from build123d import *

# Parameters (mm, degrees)
SKETCH2_W           = 35
SKETCH2_H           = 10
BOSS_EXTRUDE1_DEPTH = 4
FILLET1_R           = 2
BOSS_EXTRUDE2_DEPTH = 13


with BuildPart() as part:
    # Sketch2 → Boss-Extrude1 (new body)
    with BuildSketch(Plane.XY):
        Rectangle(SKETCH2_W, SKETCH2_H)
    extrude(amount=BOSS_EXTRUDE1_DEPTH)

    # Fillet1
    fillet1_edges = [part.edges().sort_by_distance(p)[0] for p in [
        (17.5, -5, 2),
        (-17.5, -5, 2),
        (-17.5, 5, 2),
        (17.5, 5, 2),
    ]]
    fillet(fillet1_edges, radius=FILLET1_R)

    # Sketch3 → Boss-Extrude2 (add)
    with BuildSketch(Plane.XY.offset(4)):
        with BuildLine():
            Line((-16.5, 3), (-16.5, -3))
            ThreePointArc((-16.5, -3), (-16.207106781, -3.707106781), (-15.5, -4))
            Line((-15.5, -4), (15.5, -4))
            ThreePointArc((15.5, -4), (16.207106781, -3.707106781), (16.5, -3))
            Line((16.5, -3), (16.5, 3))
            ThreePointArc((16.5, 3), (16.207106781, 3.707106781), (15.5, 4))
            Line((15.5, 4), (-15.5, 4))
            ThreePointArc((-15.5, 4), (-16.207106781, 3.707106781), (-16.5, 3))
        make_face()
    extrude(amount=BOSS_EXTRUDE2_DEPTH)


solid = part.part
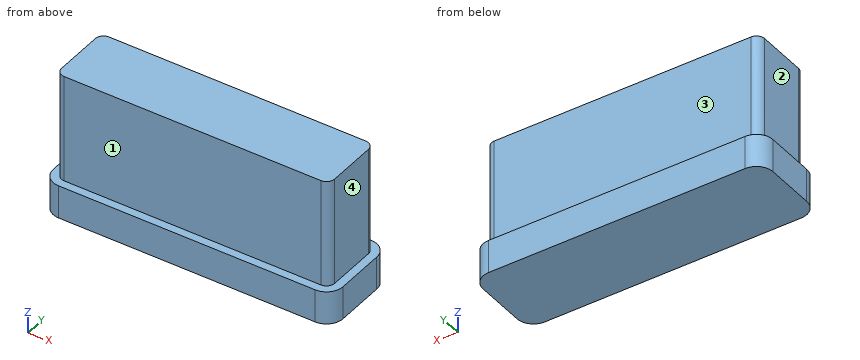
Build history of the part. All positions in model axes, mm. Face numbers are marked on the shaded views. A direction names the side the tool comes from. Round coordinates to 2 decimals unless told otherwise and drop trailing zeros. Loops run counter-clockwise (first coordinate to the right, second up) from the corner with the lowest first, then second, coordinate; pieces in that order, holes last. Notation, with made-up numbers: (80, 68.5) -> (137, 68.5) arc R26 ccw to (137, 84.5) -> close; hole circle Ø6 at (25.5, -34). An arc over 180 degrees is marked (long way). Use CSV: the item, a comma, the result in double quotes. Start each with the question number.
Q1. Saw through at A-A on x = 14. Give the cut face in (y, z), and give its area (3 significant figures).
Q2. Saw through at B-B on y = 1.5. Give the cut face in (x, z), and give its area (3 significant figures).
Q3. Drill centre lines: L1, parallel to X at y = 2, z = 12; L2, parallel to Z at x = -10, y = 4.25; L3, parallel to Y at x = -2.5, z = 15. Where is each one in solid material? Low to high.
Q4. Which spindle directions (+Z, -Z, +X, -X, +Y, -Y) get a long thin tool onto all of the face, cutting with end or side? Do the marked faces 1, 2, 3 and 4. Say none if no direction does.
Q5. Flat gauge pins, fed straight in: pin 1 Ø4 at (x, z) = (-3, 10.5) entering from +Y; pin 2 Ø4 at (x, z) = (-7.5, 7.5) entering from -Y; pin 3 Ø5 at (y, z) = (-1, 7.5) entering from +X. Where does each tip first touch, or does it go through?
Solutions:
1,outline,"(-5, 0) -> (5, 0) -> (5, 4) -> (4, 4) -> (4, 17) -> (-4, 17) -> (-4, 4) -> (-5, 4) -> close"
1,area,"144 mm^2"
2,outline,"(-17.5, 0) -> (17.5, 0) -> (17.5, 4) -> (16.5, 4) -> (16.5, 17) -> (-16.5, 17) -> (-16.5, 4) -> (-17.5, 4) -> close"
2,area,"569 mm^2"
3,L1,"x = -16.5 to 16.5"
3,L2,"z = 0 to 4"
3,L3,"y = -4 to 4"
4,face 1,"+Z, +X, -X, -Y"
4,face 2,"+Z, -X, +Y, -Y"
4,face 3,"+Z, +X, -X, +Y"
4,face 4,"+Z, +X, +Y, -Y"
5,pin 1,"stops at y = 4"
5,pin 2,"stops at y = -4"
5,pin 3,"stops at x = 16.5"
